Build history of the part. All positions in model axes, mm. A direction names the side the tool comes from. Round coordinates to 2 decimals unless told otherwise and drop trailing zeros. Loops run counter-clockwise (first coordinate to the right, second up) from the corner with the lowest first, then second, coordinate; pieces in that order, holes last. Notation, with made-up numbers: (47, -5.5) - (59, -5.5) arc R17 ccw to (59, 27.5) - close; hole circle Ø4 at (44.5, 35). An arc over 180 degrees is marked (long way). Answer as CSV lines item,"result". Start each with the question number.
```python
from build123d import *

# Parameters (mm, degrees)
SKETCH3_R           = 3.175
BOSS_EXTRUDE1_DEPTH = 3.683
CUT_SWEEP1_PITCH    = 1.27
SKETCH10_R          = 2.2225
BOSS_EXTRUDE5_DEPTH = 32.766
SKETCH9_R           = 5.08
BOSS_EXTRUDE4_DEPTH = 0.127
DOME3_FACE_RADIUS   = 5.08
DOME3_HEIGHT        = 2.38
SKETCH11_R          = 1.8415
BOSS_EXTRUDE6_DEPTH = 0.508


with BuildPart() as part:
    # Sketch3 → Boss-Extrude1 (new body)
    with BuildSketch(Plane.XY):
        Circle(SKETCH3_R)
    extrude(amount=BOSS_EXTRUDE1_DEPTH)

    # Cut-Sweep1: arcs per turn and ends read off the stored shape
    # Cut-Sweep1: the profile of Sketch5 profile screwed along a left-hand helix through 4 turns, 8 arcs to a turn; built about Z, then put on its axis
    cut_sweep1_z = Axis((0, 0, 0), (0, 0, 1))
    cut_sweep1_corners = [(2.54, 0, -1.397), (3.1753, 0, -1.763790626), (3.1753, 0, -0.776209374), (2.54, 0, -1.143)]
    with BuildLine(mode=Mode.PRIVATE) as cut_sweep1_profile:
        Line(cut_sweep1_corners[0], cut_sweep1_corners[1])
        Line(cut_sweep1_corners[1], cut_sweep1_corners[2])
        Line(cut_sweep1_corners[2], cut_sweep1_corners[3])
        Line(cut_sweep1_corners[3], cut_sweep1_corners[0])
    cut_sweep1_cap = Face(cut_sweep1_profile.wire())
    cut_sweep1_turn_angles = [0, -22.5, -45, -67.5, -90, -112.5, -135, -157.5, -180, -202.5, -225, -247.5, -270, -292.5, -315, -337.5, -360]
    cut_sweep1_turn_weights = [1, 0.9238795325112867, 1, 0.9238795325112867, 1, 0.9238795325112867, 1, 0.9238795325112867, 1, 0.9238795325112867, 1, 0.9238795325112867, 1, 0.9238795325112867, 1, 0.9238795325112867, 1]
    cut_sweep1_turn_rails = [Edge.make_bspline([Vector(p[0], p[1], 0).rotate(cut_sweep1_z, cut_sweep1_turn_angles[k]) / cut_sweep1_turn_weights[k] + Vector(0, 0, p[2] + -CUT_SWEEP1_PITCH * cut_sweep1_turn_angles[k] / 360) for k in range(17)], [0, 0, 0, 1, 1, 2, 2, 3, 3, 4, 4, 5, 5, 6, 6, 7, 7, 8, 8, 8], 2, cut_sweep1_turn_weights) for p in cut_sweep1_corners]
    cut_sweep1_turn_sides = [Face.make_surface_from_curves(cut_sweep1_turn_rails[p[0]], cut_sweep1_turn_rails[p[1]]) for p in [(0, 1), (1, 2), (2, 3), (3, 0)]]
    cut_sweep1 = Plane(origin=(0, 0, 0), x_dir=(0, 1, 0), z_dir=(0, 0, 1)) * Solid(Shell([*[p.moved(Location((0, 0, CUT_SWEEP1_PITCH * i))) for i in range(4) for p in cut_sweep1_turn_sides], cut_sweep1_cap, cut_sweep1_cap.rotate(cut_sweep1_z, -1440).moved(Location((0, 0, -CUT_SWEEP1_PITCH * -1440 / 360)))]))
    add(cut_sweep1, mode=Mode.SUBTRACT)

    # Sketch10 → Boss-Extrude5 (add)
    with BuildSketch(Plane.XY.offset(3.683)):
        Circle(SKETCH10_R)
    extrude(amount=BOSS_EXTRUDE5_DEPTH)

    # Sketch9 → Boss-Extrude4 (add)
    with BuildSketch(Plane.XY):
        Circle(SKETCH9_R)
    extrude(amount=-BOSS_EXTRUDE4_DEPTH)

    # Dome3: a dome of height H over a round flat face of radius A is a cap of a sphere of radius (A * A + H * H) / (2 * H)
    dome3_r = (DOME3_FACE_RADIUS * DOME3_FACE_RADIUS + DOME3_HEIGHT * DOME3_HEIGHT) / (2 * DOME3_HEIGHT)
    dome3_base = Plane((0, 0, -0.127), z_dir=(0, 0, -1))
    with Locations(dome3_base.offset(DOME3_HEIGHT - dome3_r)):
        dome3_ball = Sphere(dome3_r, mode=Mode.PRIVATE)
    add(split(dome3_ball, bisect_by=dome3_base, keep=Keep.TOP, mode=Mode.PRIVATE))

    # Sketch11 → Boss-Extrude6 (add)
    with BuildSketch(Plane.XY.offset(36.449)):
        Circle(SKETCH11_R)
    extrude(amount=BOSS_EXTRUDE6_DEPTH)


solid = part.part
```
Q1. Wall check: probe 1 along Z at (x, y) = (0, 1); probe 2 along X at (y, z) = (0.5, 13.5); probe 3 along Z at (x, y) = (3, -1.25). Give the ranges that are in metal, low to high. Write a range as [from, to].
Q2. Pin check, flat tips, straight feed: pin 1 Ø5 at (y, z) = (-2.5, 16) entering from +X; pin 2 Ø1.5 at (x, y) = (-1, -3.5) entering from -Z; pin 3 Ø1.5 at (y, z) = (2, 28.5) entering from +X. Stop position of each tip, or through.
Q3. Band-saw the part on B-B, the plane x = 3.75. List the corners of the cut face in (y, z), then the cut area to 3 significant figures.
Q4. Band-saw the part on C-C, the plane y = 4.5. List the corners of the cut face in (x, z), then the cut area to 3 significant figures.
Q5. Band-saw the part on A-A, the plane z = 31. List the corners of the cut face in (x, y) (1 decimal).
Q6. Tool access for faces 1 (the cylindrical face through (0.85, -1.634, 36.699)), 2 (the flat face through (0, 0, 36.957)): list every direction of +Z, -Z, +X, -X, +Y, -Y with a clear straight run to the whole face (end or side of a thin tool).
Reported:
1,probe 1,"z = [-2.43, 36.96]"
1,probe 2,"x = [-2.17, 2.17]"
1,probe 3,"z = [-1.65, 0]"
2,pin 1,"stops at x = 2.22"
2,pin 2,"stops at z = -1.84"
2,pin 3,"stops at x = 1.84"
3,outline,"(-3.43, -0.13) arc R5.45 ccw to (3.43, -0.13) - (3.43, 0) - (-3.43, 0) - close"
3,area,"6.55 mm2"
4,outline,"(-2.36, -0.13) arc R4.84 ccw to (2.36, -0.13) - (2.36, 0) - (-2.36, 0) - close"
4,area,"2.55 mm2"
5,outline,"circle Ø4.4 at (0, 0)"
6,face 1,"+Z"
6,face 2,"+Z, +X, -X, +Y, -Y"
